For this review, take the finished solid that the model builds, in its own axes (mm). Face numbers are marked on the shaded views. A direction names the side the tool comes from. Give positions to 0.01 mm unless a question says otherwise; leave off trailing zeros. Write each loop counter-clockwise with the first axis right and the second up, starting at its lowest first coordinate (ties: lowest second). Pieces come first, ordered by that corner, then holes.
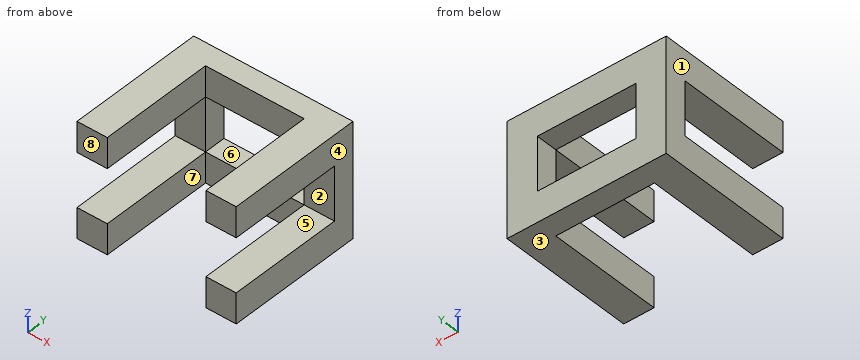
from build123d import *

# Parameters (mm, degrees)
SKETCH1_W           = 36.8
SKETCH1_H           = 26.4
SKETCH1_W_2         = 22.8
SKETCH1_H_2         = 12.4
BOSS_EXTRUDE1_DEPTH = 5
SKETCH2_W           = 7
SKETCH2_H           = 7
BOSS_EXTRUDE2_DEPTH = 26.5


with BuildPart() as part:
    # Sketch1 → Boss-Extrude1 (new body)
    with BuildSketch(Plane(origin=(0, 0, 0), x_dir=(1, 0, 0), z_dir=(0, 1, 0))):
        with Locations((1.98028169, 1.052112676)):
            Rectangle(SKETCH1_W, SKETCH1_H)
        with Locations((1.98028169, 1.052112676)):
            Rectangle(SKETCH1_W_2, SKETCH1_H_2, mode=Mode.SUBTRACT)
    extrude(amount=BOSS_EXTRUDE1_DEPTH)

    # Sketch2 → Boss-Extrude2 (add)
    with BuildSketch(Plane.XZ):
        with Locations((16.88028169, -10.752112676)):
            Rectangle(SKETCH2_W, SKETCH2_H)
        with Locations((-12.91971831, -10.752112676)):
            Rectangle(SKETCH2_W, SKETCH2_H)
        with Locations((-12.91971831, 8.647887324)):
            Rectangle(SKETCH2_W, SKETCH2_H)
        with Locations((16.88028169, 8.647887324)):
            Rectangle(SKETCH2_W, SKETCH2_H)
    extrude(amount=BOSS_EXTRUDE2_DEPTH)


solid = part.part
(1) We need section A-A (x = -2). Write out the cut boundary in (y, z).
(2) Tool access review of the marked faces 4, 5, 6, 7 and 8: name each direction out of +Z, -Z, +X, -X, +Y, -Y from which nothing blocks a thin tool from reaching the whole face with its end or side.
(3) We need section C-C (z = 1). Write out the cut boundary in (x, y).
(4) We need section D-D (y = -11). Write out the cut boundary in (x, z).
(5) We need section B-B (y = 3). Write out the cut boundary in (x, z), and give its area (3 significant figures).
(6) Clearance check with a flat-ended pin moving along its axis: pin 1 Ø3.5 at (x, z) = (0.5, -11.5) entering from -Y. State where the tip first meets the part, or that it passes through.
(7) For L1, parallel to X at y = -3, z = 6.25; L2, parallel to Z at x = -10, y = -22; L3, parallel to Y at x = 15.5, z = -4.25, list the stretches that pass through material, from the lowest coordinate up.
(8) The part is to be moulded in two halves that separate along Z. For the marked faces 1, 2 and 3, say which applies: +Z half, -Z half, draft (parallel to the pull), parting line (faces both ways), or undercut.
The answers:
1. outline: (0, -14.25) - (5, -14.25) - (5, -7.25) - (0, -7.25) - close; (0, 5.15) - (5, 5.15) - (5, 12.15) - (0, 12.15) - close
2. face 4: +Z, -Z, +X, +Y, -Y
2. face 5: +X, -X, -Y
2. face 6: +Y, -Y
2. face 7: +Z, -Z, -Y
2. face 8: +Z, -Z, +X, -X, -Y
3. outline: (-16.42, 0) - (-9.42, 0) - (-9.42, 5) - (-16.42, 5) - close; (13.38, 0) - (20.38, 0) - (20.38, 5) - (13.38, 5) - close
4. outline: (-16.42, -14.25) - (-9.42, -14.25) - (-9.42, -7.25) - (-16.42, -7.25) - close; (-16.42, 5.15) - (-9.42, 5.15) - (-9.42, 12.15) - (-16.42, 12.15) - close; (13.38, -14.25) - (20.38, -14.25) - (20.38, -7.25) - (13.38, -7.25) - close; (13.38, 5.15) - (20.38, 5.15) - (20.38, 12.15) - (13.38, 12.15) - close
5. outline: (-16.42, -14.25) - (20.38, -14.25) - (20.38, 12.15) - (-16.42, 12.15) - close; hole (-9.42, -7.25) - (13.38, -7.25) - (13.38, 5.15) - (-9.42, 5.15) - close
5. area: 689 mm2
6. pin 1: stops at y = 0
7. L1: x = -16.42 to -9.42, 13.38 to 20.38
7. L2: z = -14.25 to -7.25, 5.15 to 12.15
7. L3: y = 0 to 5
8. face 1: draft
8. face 2: undercut
8. face 3: -Z half
